Geometry: see drawing. Coordinates: mm, zero at the bounding-box minimum. A direction names the side the tool comes from. Round coordinates to 2 decimals unless told otherwise and drop trailing zeros. Loops run counter-clockwise (first coordinate to the right, second up) from the corner with the lowest first, then second, coordinate; pieces in that order, holes last.
(1) Section A-A, the plane y = 4.2. Return the cut outline in (x, z).
(2) Section D-D, the plane x = 9.5. Return the cut outline in (y, z).
(3) Section C-C, the plane z = 6.5. Return the cut outline in (x, y), plus the area to 3 significant figures.
(4) Material intervals for probe 1 along X at (y, z) = (3.45, 6.5); probe 2 along Z at (x, y) = (4, 4.55), sorted ascending.
(5) Set-up query: the marked faces 1 and 2. Return all of +Z, -Z, +X, -X, +Y, -Y with unobstructed straight access to the full face (end or side cutting, diameter ignored); none if empty.
(6) Section B-B, the plane x = 6.5. Return the cut outline in (y, z).
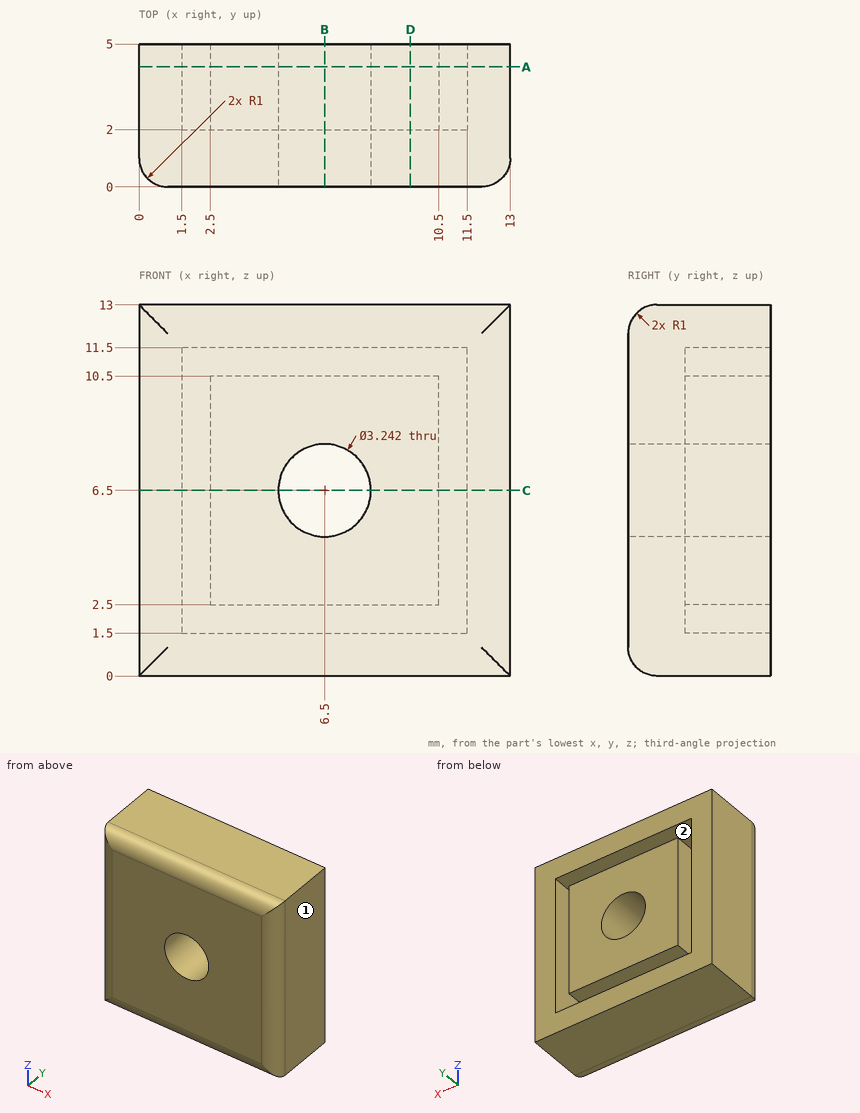
Output values:
1. outline: (0, 0) - (13, 0) - (13, 13) - (0, 13) - close; (2.5, 2.5) - (10.5, 2.5) - (10.5, 10.5) - (2.5, 10.5) - close; hole (1.5, 1.5) - (11.5, 1.5) - (11.5, 11.5) - (1.5, 11.5) - close; hole circle Ø3.24 at (6.5, 6.5)
2. outline: (0, 1) arc R1 ccw to (1, 0) - (5, 0) - (5, 1.5) - (2, 1.5) - (2, 2.5) - (5, 2.5) - (5, 10.5) - (2, 10.5) - (2, 11.5) - (5, 11.5) - (5, 13) - (1, 13) arc R1 ccw to (0, 12) - close
3. outline: (0, 1) arc R1 ccw to (1, 0) - (4.88, 0) - (4.88, 5) - (2.5, 5) - (2.5, 2) - (1.5, 2) - (1.5, 5) - (0, 5) - close; (8.12, 0) - (12, 0) arc R1 ccw to (13, 1) - (13, 5) - (11.5, 5) - (11.5, 2) - (10.5, 2) - (10.5, 5) - (8.12, 5) - close
3. area: 42.4 mm2
4. probe 1: x = 0 to 1.5, 2.5 to 4.88, 8.12 to 10.5, 11.5 to 13
4. probe 2: z = 0 to 1.5, 2.5 to 10.5, 11.5 to 13
5. face 1: +Z, -Z, +X, +Y, -Y
5. face 2: +Y
6. outline: (0, 1) arc R1 ccw to (1, 0) - (5, 0) - (5, 1.5) - (2, 1.5) - (2, 2.5) - (5, 2.5) - (5, 4.88) - (0, 4.88) - close; (0, 8.12) - (5, 8.12) - (5, 10.5) - (2, 10.5) - (2, 11.5) - (5, 11.5) - (5, 13) - (1, 13) arc R1 ccw to (0, 12) - close
